```python
from build123d import *

# Parameters (mm, degrees)
SKETCH1_W            = 30
SKETCH1_H            = 30
BOSS_EXTRUDE1_DEPTH  = 4
SKETCH3_W            = 30
SKETCH3_H            = 5
BOSS_EXTRUDE2_DEPTH  = 24
SKETCH4_W            = 40.2
SKETCH4_H            = 5
BOSS_EXTRUDE3_DEPTH  = 5
SKETCH5_W            = 5
SKETCH5_H            = 24.2
BOSS_EXTRUDE4_DEPTH  = 8.5
LPATTERN1_COUNT      = 2
LPATTERN1_PITCH      = 48.7
M4_CLEARANCE_HOLE1_D = 4.5


with BuildPart() as part:
    # Sketch1 → Boss-Extrude1 (new body)
    with BuildSketch(Plane(origin=(0, 0, 0), x_dir=(0, 0, -1), z_dir=(1, 0, 0))):
        with Locations((15, 15)):
            Rectangle(SKETCH1_W, SKETCH1_H)
    extrude(amount=BOSS_EXTRUDE1_DEPTH)

    # Sketch3 → Boss-Extrude2 (add)
    with BuildSketch(Plane(origin=(4, 0, 0), x_dir=(0, 0, -1), z_dir=(1, 0, 0))):
        with Locations((15, 27.5)):
            Rectangle(SKETCH3_W, SKETCH3_H)
    extrude(amount=BOSS_EXTRUDE2_DEPTH)

    # Sketch4 → Boss-Extrude3 (add)
    with BuildSketch(Plane(origin=(28, 0, 0), x_dir=(0, 0, -1), z_dir=(1, 0, 0))):
        with Locations((15, 27.5)):
            Rectangle(SKETCH4_W, SKETCH4_H)
    extrude(amount=BOSS_EXTRUDE3_DEPTH)

    # Sketch5 → Boss-Extrude4 (add)
    with BuildSketch(Plane.XY.offset(5.1)):
        with Locations((30.5, 17.9)):
            Rectangle(SKETCH5_W, SKETCH5_H)
    boss_extrude4 = extrude(amount=BOSS_EXTRUDE4_DEPTH)

    # LPattern1: Boss-Extrude4 ×2
    with Locations(*[(0, 0, -i * LPATTERN1_PITCH) for i in range(1, LPATTERN1_COUNT)]):
        add(boss_extrude4)

    # M4 Clearance Hole1 (through all)
    with Locations(Plane(origin=(33, 0, 0), x_dir=(0, 0, -1), z_dir=(1, 0, 0))):
        with Locations((-9.35, 20.3), (-9.35, 9.9), (39.35, 20.3), (39.35, 9.9)):
            Hole(M4_CLEARANCE_HOLE1_D / 2)


solid = part.part
```
Work out the finished part from the listing and answer in its coordinate system (mm). A direction names the side the tool comes from. Round coordinates to 2 decimals unless told otherwise and drop trailing zeros. Loops run counter-clockwise (first coordinate to the right, second up) from the corner with the lowest first, then second, coordinate; pieces in that order, holes last. Notation, with made-up numbers: M 33,20 L 41,20 A10 cw 41,25 Z; hole C 57,59 d8. An arc over 180 degrees is marked long. Use CSV: the item, a comma, the result in double quotes.
Q1. Section C-C, the plane y = 15.25 is taken. Determine the outline of the cut face in (x, z).
Determined:
outline,"M 0,-30 L 4,-30 L 4,0 L 0,0 Z; M 28,-43.6 L 33,-43.6 L 33,-35.1 L 28,-35.1 Z; M 28,5.1 L 33,5.1 L 33,13.6 L 28,13.6 Z"
Q2. Section B-B, the plane z = 9.35 is taken. Determine the outline of the cut face in (x, y).
Determined:
outline,"M 28,5.8 L 33,5.8 L 33,7.65 L 28,7.65 Z; M 28,12.15 L 33,12.15 L 33,18.05 L 28,18.05 Z; M 28,22.55 L 33,22.55 L 33,30 L 28,30 Z"
Q3. A tool of negligible diameter and unlimited length cuts with its end or side. For faces 4 (the flat face through (28, 18, 8)), 5 (the flat face through (18, 25, -15)), 6 (the flat face through (28, 18, -38)), 7 (the flat face through (4, 13, -15)), 8 (the flat face through (30, 16, -35.1)), from which of +Z, -Z, +X, -X, +Y, -Y can it reach the whole face along a straight path? Write none if from no direction.
Determined:
face 4,"+Z, -X, +Y, -Y"
face 5,"+X, -Y"
face 6,"-Z, -X, +Y, -Y"
face 7,"+Z, -Z, +X, -Y"
face 8,"+X, -X, -Y"
Q4. Section D-D, the plane y = 26 is taken. Determine the outline of the cut face in (x, z), then the cut area to 3 significant figures.
Determined:
outline,"M 0,-30 L 28,-30 L 28,-43.6 L 33,-43.6 L 33,13.6 L 28,13.6 L 28,0 L 0,0 Z"
area,"1,130 mm2"
Q5. Consider L1, parallel to Y at x = 29.45, z = 9.35; L2, parallel to X at y = 14.25, z = -15; L3, parallel to X at y = 27.25, z = 6. Determine where each line is inside the solid, lowest interval first.
Determined:
L1,"5.8 to 7.65, 12.15 to 18.05, 22.55 to 30"
L2,"0 to 4"
L3,"28 to 33"
Q6. Each of these flat-tipped pins is pushed along its axis until it touches: pin 1 (5.5 mm diameter, centred on x = 30, z = 10, fed in from -Y); pin 2 (3 mm diameter, centred on y = 11.5, z = -1, fed in from +X); pin 3 (6 mm diameter, centred on y = 14, z = 7.5, fed in from -X). Where does it stop, or does it pass through?
Determined:
pin 1,"y = 5.8"
pin 2,"x = 4"
pin 3,"x = 28"
Q7. The mould has two halves that part along Z. Classify faces 1 (the flat face through (30, 18, 13.6)), 2 (the flat face through (30, 5.8, -39)), 3 (the cylindrical face through (30.47, 12.13, 9.06)): pulls with the +Z half, pulls with the -Z half, needs draft (parallel to the pull), parting line crosses it, or undercut.
Determined:
face 1,"pulls with the +Z half"
face 2,"needs draft"
face 3,"undercut"
Q8. Section A-A, the plane y = 20.3 is taken. Determine the outline of the cut face in (x, z), then the cut area to 3 significant figures.
Determined:
outline,"M 0,-30 L 4,-30 L 4,0 L 0,0 Z; M 28,-43.6 L 33,-43.6 L 33,-41.6 L 28,-41.6 Z; M 28,-37.1 L 33,-37.1 L 33,-35.1 L 28,-35.1 Z; M 28,5.1 L 33,5.1 L 33,7.1 L 28,7.1 Z; M 28,11.6 L 33,11.6 L 33,13.6 L 28,13.6 Z"
area,"160 mm2"
